Model file for the job. Use its own axes, mm. Face numbers are marked on the shaded views. A direction names the side the tool comes from. Coordinates: 2 decimals unless noted, no trailing zeros. Order: outer loops, then holes, each group sorted by start corner. A loop starts at its lowest first (then second) coordinate and runs counter-clockwise, first axis right, second up. Notation, with made-up numbers: M 85,36.25 L 113,36.25 A12 ccw 113,43.25 Z; hole C -14.75,86 d4. An arc over 180 degrees is marked long. Return JSON: item names as keys, results as strings.
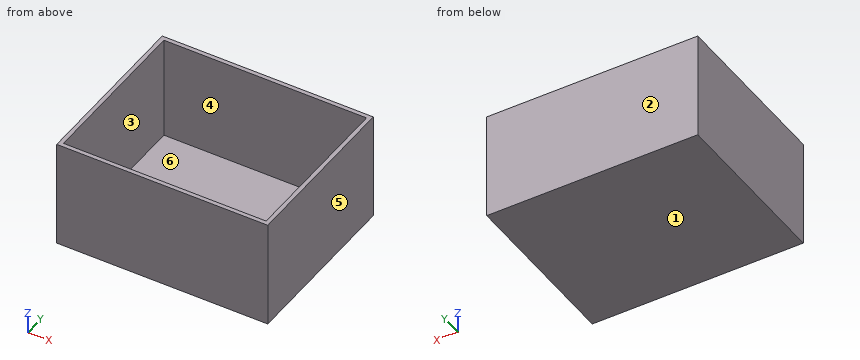
```python
from build123d import *

# Parameters (mm, degrees)
SHEET_EXTRUDE_1_2_DEPTH = 50
SKETCH_1_2_W            = 97.399040294
SKETCH_1_2_H            = 78.98176722
THICKEN_1_T1            = 2


with BuildPart() as body_1:
    # Sheet Extrude 1: a surface, the sketch's curves swept straight by 50 mm
    with BuildLine(Plane.XY, mode=Mode.PRIVATE) as sheet_extrude_1_2_path:
        Line((-42.324310237, 40.376329431), (55.074730057, 40.376329431))
        Line((55.074730057, 40.376329431), (55.074730057, -38.605437789))
        Line((55.074730057, -38.605437789), (-42.324310237, -38.605437789))
        Line((-42.324310237, -38.605437789), (-42.324310237, 40.376329431))
    sheet_extrude_1_2 = Shell.extrude(sheet_extrude_1_2_path.wire(), (0 * SHEET_EXTRUDE_1_2_DEPTH, 0 * SHEET_EXTRUDE_1_2_DEPTH, 1 * SHEET_EXTRUDE_1_2_DEPTH))
    # Эскиз1<2> → Sheet Fill 1: a flat surface bounded by the sketch
    with BuildSketch(Plane.XY, mode=Mode.PRIVATE) as sheet_fill_1_3_region:
        with Locations((6.37520991, 0.885445821)):
            Rectangle(SKETCH_1_2_W, SKETCH_1_2_H)
    sheet_fill_1_3 = sheet_fill_1_3_region.sketch.faces()[0]
    # Knit 1: the surfaces knitted into one
    knit_1_1 = Shell(Face.sew_faces(sheet_extrude_1_2.faces() + sheet_fill_1_3.faces())[0])
    add(Solid.thicken(knit_1_1, THICKEN_1_T1))


solid = body_1.part
```
Item 1: Wall check: line 1 (X direction, y = 0.5, z = 5.5); line 2 (Y direction, x = 31.5, z = 35); line 3 (Z direction, x = -10, y = -28). Give the ranges that are in metal, low to high.
Check result:
{"line 1": "x = -44.32 to -42.32, 55.07 to 57.07", "line 2": "y = -40.61 to -38.61, 40.38 to 42.38", "line 3": "z = -2 to 0"}
Item 2: Saw through at B-B (z = 33). Write the cut outline in (x, y), and give its area (3 significant figures).
Check result:
{"outline": "M -44.32,-40.61 L 57.07,-40.61 L 57.07,42.38 L -44.32,42.38 Z; hole M -42.32,-38.61 L 55.07,-38.61 L 55.07,40.38 L -42.32,40.38 Z", "area": "722 mm2"}
Item 3: 3-axis set-ups, long thin cutter, end or side, ignore diameter. For the marked faces 5 and 6: which of +Z, -Z, +X, -X, +Y, -Y reach the whole face in a straight line?
Check result:
{"face 5": "+Z, -Z, +X, +Y, -Y", "face 6": "+Z"}
Item 4: Saw through at A-A (y = -20.5). Write the cut outline in (x, z), and give its area (3 significant figures).
Check result:
{"outline": "M -44.32,-2 L 57.07,-2 L 57.07,50 L 55.07,50 L 55.07,0 L -42.32,0 L -42.32,50 L -44.32,50 Z", "area": "403 mm2"}
Item 5: Saw through at C-C (x = -35.5). Write the cut outline in (y, z).
Check result:
{"outline": "M -40.61,-2 L 42.38,-2 L 42.38,50 L 40.38,50 L 40.38,0 L -38.61,0 L -38.61,50 L -40.61,50 Z"}
Item 6: Pull direction Y, two halves, no side cores. Call the marked faces 1, 2, 3 and 4: +Y half, -Y half, draft (parallel to the pull), parting line (faces both ways), or undercut.
Check result:
{"face 1": "draft", "face 2": "+Y half", "face 3": "undercut", "face 4": "undercut"}
Item 7: Drop a flat-ended pin along its axis: pin 1 Ø1 at (x, y) = (-27, 1.5) entering from +Z. Give the stop position or say it passes through.
Check result:
{"pin 1": "stops at z = 0"}
